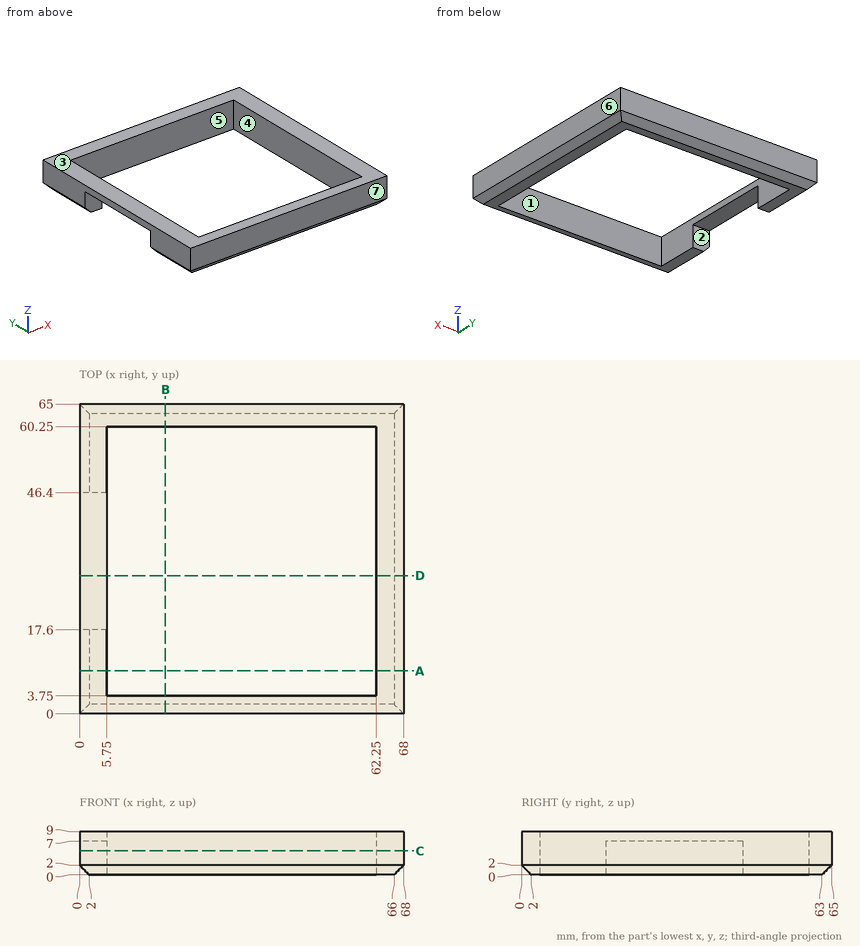
Design review of the part shown in the three views and the two pictorial views. Dimensions are in mm from the part's minimum x, y and z. A direction names the side the tool comes from. Give positions to 0.01 mm unless a question says otherwise; leave off trailing zeros. Loops run counter-clockwise (first coordinate to the right, second up) from the corner with the lowest first, then second, coordinate; pieces in that order, holes last. Notation, with made-up numbers: (78, 82) - (121, 82) arc R17 ccw to (121, 108) - close; hole circle Ø8 at (11.5, -35). An arc over 180 degrees is marked (long way). Use CSV: the item, a comma, the result in double quotes. Start each with the question number.
1. Wall thickness on L1, parallel to X at y = 49, z = 5.5; L2, parallel to Y at x = 53, z = 3: over which ranges is each line inside the solid? List them lowest first.
2. Add section B-B (x = 18). State the section outline as (y, z) points, plus the area to 3 significant figures.
3. Insertion check: P1, Ø12, axis at x = 56, y = 55.5, coming from the -Z side; P2, Ø4, axis at y = 38.5, z = 1.5, coming from the -X side; P3, Ø1.7, axis at x = 1.5, y = 35, coming from the -Z side. Each pin has a flat end and moves straight along its axis. Give the tip position at first contact, or say it passes through.
4. Draft analysis for pull direction Y (two halves, no side actions). For the marked faces 4, 5, 6 and 7, state which applies: released by +Y, released by -Y, zero draft, split by the parting line, or undercut.
5. Add section D-D (y = 29). State the section outline as (x, z) points, plus the area to 4 significant figures.
6. Add section A-A (y = 9). State the section outline as (x, z) points.
7. Machinability: for the marked faces 1, 2 and 3, which of the approach directions +Z, -Z, +X, -X, +Y, -Y give a long, thin tool a straight path to every point of the face, cutting with its end or side? Answer none if there is none.
8. Add section C-C (z = 5). State the section outline as (x, y) points, plus the area to 3 significant figures.
Results found:
1,L1,"x = 0 to 5.75, 62.25 to 68"
1,L2,"y = 0 to 3.75, 60.25 to 65"
2,outline,"(0, 2) - (2, 0) - (3.75, 0) - (3.75, 9) - (0, 9) - close; (60.25, 0) - (63, 0) - (65, 2) - (65, 9) - (60.25, 9) - close"
2,area,"72.5 mm²"
3,P1,"stops at z = 0"
3,P2,"stops at x = 62.25"
3,P3,"stops at z = 7"
4,face 4,"undercut"
4,face 5,"undercut"
4,face 6,"zero draft"
4,face 7,"released by -Y"
5,outline,"(0, 7) - (5.75, 7) - (5.75, 9) - (0, 9) - close; (62.25, 0) - (66, 0) - (68, 2) - (68, 9) - (62.25, 9) - close"
5,area,"61.25 mm²"
6,outline,"(0, 2) - (2, 0) - (5.75, 0) - (5.75, 9) - (0, 9) - close; (62.25, 0) - (66, 0) - (68, 2) - (68, 9) - (62.25, 9) - close"
7,face 1,"+Z, -Z"
7,face 2,"-Z, -X"
7,face 3,"+Z, +X, -X, +Y, -Y"
8,outline,"(0, 0) - (68, 0) - (68, 65) - (0, 65) - (0, 46.4) - (5.75, 46.4) - (5.75, 60.25) - (62.25, 60.25) - (62.25, 3.75) - (5.75, 3.75) - (5.75, 17.6) - (0, 17.6) - close"
8,area,"1,060 mm²"
